```python
from build123d import *

# Parameters (mm, degrees)
BOSS_EXTRUDE1_DEPTH            = 40
SKETCH2_W                      = 40
SKETCH2_H                      = 30
BOSS_EXTRUDE2_DEPTH            = 20
BOSS_EXTRUDE3_DEPTH            = 30
CUT_EXTRUDE1_DEPTH             = 30
SKETCH5_W                      = 70
SKETCH5_H                      = 40
BOSS_EXTRUDE4_DEPTH            = 10
SKETCH6_W                      = 20
SKETCH6_H                      = 20
CUT_EXTRUDE2_DEPTH             = 41
F_10_0_10_DIAMETER_HOLE1_D     = 10
F_10_0_10_DIAMETER_HOLE1_DEPTH = 40
FILLET1_R                      = 20


with BuildPart() as part:
    # Sketch1 → Boss-Extrude1 (new body)
    with BuildSketch(Plane(origin=(0, 0, 0), x_dir=(0, -1, 0), z_dir=(-1, 0, 0))):
        Polygon((-10, -10), (-40, -20), (-10, -20), align=None)
    extrude(amount=-BOSS_EXTRUDE1_DEPTH)

    # Sketch2 → Boss-Extrude2 (add)
    with BuildSketch(Plane(origin=(0, 0, -20), x_dir=(-1, 0, 0), z_dir=(0, 0, -1))):
        with Locations((-20, 25)):
            Rectangle(SKETCH2_W, SKETCH2_H)
    extrude(amount=BOSS_EXTRUDE2_DEPTH)

    # Sketch3 → Boss-Extrude3 (add)
    with BuildSketch(Plane(origin=(40, 0, 0), x_dir=(0, 0, -1), z_dir=(1, 0, 0))):
        Polygon((40, 10), (0, 10), (20, 40), (40, 40), align=None)
    extrude(amount=BOSS_EXTRUDE3_DEPTH)

    # Sketch4 → Cut-Extrude1 (cut)
    with BuildSketch(Plane(origin=(70, 0, 0), x_dir=(0, 0, -1), z_dir=(1, 0, 0))):
        Polygon((20, 40), (0, 10), (30, 10), (30, 30), (40, 30), (40, 40), align=None)
    extrude(amount=-CUT_EXTRUDE1_DEPTH, mode=Mode.SUBTRACT)

    # Sketch5 → Boss-Extrude4 (add)
    with BuildSketch(Plane.XZ.offset(-10)):
        with Locations((35, -20)):
            Rectangle(SKETCH5_W, SKETCH5_H)
    extrude(amount=BOSS_EXTRUDE4_DEPTH)

    # Sketch6 → Cut-Extrude2 (cut, through all)
    with BuildSketch(Plane(origin=(0, 0, -40), x_dir=(-1, 0, 0), z_dir=(0, 0, -1))):
        with Locations((-20, 30)):
            Rectangle(SKETCH6_W, SKETCH6_H)
    extrude(amount=-CUT_EXTRUDE2_DEPTH, mode=Mode.SUBTRACT)

    # Ø10.0 (10) Diameter Hole1
    with Locations(Plane(origin=(0, 0, 0), x_dir=(-1, 0, 0), z_dir=(0, -1, 0))):
        with Locations((-55, 15)):
            Hole(F_10_0_10_DIAMETER_HOLE1_D / 2, depth=F_10_0_10_DIAMETER_HOLE1_DEPTH)

    # Fillet1
    fillet1_edges = [part.edges().sort_by_distance(p)[0] for p in [
        (70, 30, -35),
    ]]
    fillet(fillet1_edges, radius=FILLET1_R)


solid = part.part
```
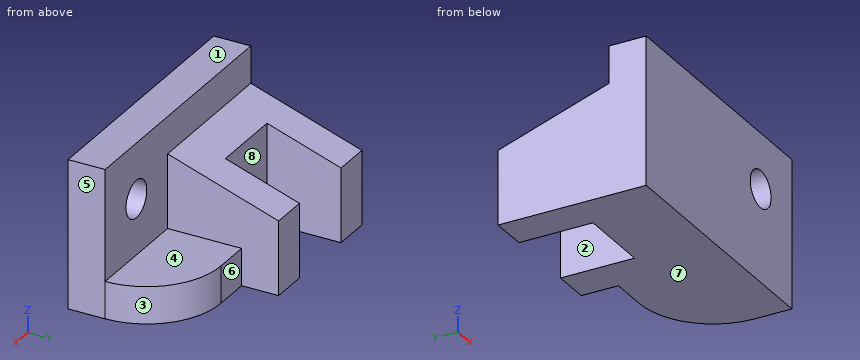
Geometry check sheet. Reference: the model listing, model coordinates, mm. Face numbers are marked on the shaded views. A direction names the side the tool comes from. Give positions to 0.01 mm unless a question says otherwise; leave off trailing zeros. Write each loop counter-clockwise with the first axis right and the second up, starting at its lowest first coordinate (ties: lowest second). Pieces come first, ordered by that corner, then holes.
1) Section check A-A, the plane z = -15. Record the boundary of the cut face in (x, y), and give its area (3 significant figures).
2) Material ranges on L1, parallel to Z at x = 55, y = 3; L2, parallel to X at y = 34, z = -35.5; L3, parallel to Y at x = 67.5, z = -26.5, recorded low to high.
3) Section check C-C, the plane z = -35.5. Record the boundary of the cut face in (x, y), and give its area (3 significant figures).
4) Release check for a two-part mould opening along X. For the marked faces 1, 2 and 3 record: pulls with the +X half, pulls with the -X half, needs draft (parallel to the pull), parting line crosses it, or undercut.
5) Section check D-D, the plane y = 3.5. Record the boundary of the cut face in (x, z).
6) Access from +Z, -Z, +X, -X, +Y, -Y to the whole of each face (thin tool, end or side, straight path). Record for the marked faces 4, 5, 6, 7 and 8.
7) Section check B-B, the plane y = 22. Record the boundary of the cut face in (x, z).
8) Gauge pin test, flat ends, axial feed: pin 1 (1 mm diameter, centred on x = 29, y = 28, fed in from +Z); pin 2 (5 mm diameter, centred on y = 15.5, z = -23.5, fed in from +X); pin 3 (9 mm diameter, centred on x = 19.5, z = -13, fed in from +Y); pin 4 (16 mm diameter, centred on y = 25.5, z = -32.5, fed in from +X). Record the tip position at first contact, or that the pin passes through.
Computed:
1. outline: (0, 0) - (50, 0) - (50, 10) - (40, 10) - (40, 25) - (30, 25) - (30, 20) - (10, 20) - (10, 25) - (0, 25) - close; (60, 0) - (70, 0) - (70, 10) - (60, 10) - close
1. area: 1,100 mm2
2. L1: z = -40 to -20, -10 to 0
2. L2: x = 0 to 10, 30 to 40
2. L3: y = 0 to 10
3. outline: (0, 0) - (70, 0) - (70, 10) arc R20 ccw to (50, 30) - (40, 30) - (40, 40) - (30, 40) - (30, 20) - (10, 20) - (10, 40) - (0, 40) - close
3. area: 2,010 mm2
4. face 1: needs draft
4. face 2: undercut
4. face 3: pulls with the +X half
5. outline: (0, -40) - (70, -40) - (70, 0) - (0, 0) - close; hole circle Ø10 at (55, -15)
6. face 4: +Z, +X, +Y
6. face 5: +Z, -Z, +X, +Y, -Y
6. face 6: +Z, -Z, +X, +Y
6. face 7: -Z, +X, -X, +Y, -Y
6. face 8: +Z, -Z, +Y
7. outline: (0, -40) - (10, -40) - (10, -14) - (0, -14) - close; (30, -40) - (66, -40) - (66, -30) - (40, -30) - (40, -14) - (30, -14) - close
8. pin 1: passes through
8. pin 2: stops at x = 40
8. pin 3: stops at y = 20
8. pin 4: stops at x = 68.54
